Here's how the part is built. I have some questions about the finished solid (model axes, mm). Give positions to 0.01 mm unless a question says otherwise; leave off trailing zeros. Loops run counter-clockwise (first coordinate to the right, second up) from the corner with the lowest first, then second, coordinate; pieces in that order, holes last.
Q1. If we section it at A-A (z = -1.7): Please give me the cut outline in (x, y) (1 decimal), plus the area to 3 significant figures.
Q2. I need wall thicknesses on line 1 (Y direction, x = 10, z = -2.2); line 2 (X direction, y = 135.25, z = -1.4); line 3 (Y direction, x = 31.5, z = -3). Which ranges of each line are inside material? Lowest first, please.
Q3. If we section it at C-C (x = 140.5): Please give me the cut outline in (y, z) (3 decimals).
Q4. If we section it at B-B (x = 26.5): Please give me the cut outline in (y, z) (3 decimals).
from build123d import *

# Parameters (mm, degrees)
SKETCH1_R           = 0.635
BOSS_EXTRUDE1_DEPTH = 3.175


with BuildPart() as part:
    # Sketch1 → Boss-Extrude1 (new body)
    with BuildSketch(Plane.XY):
        Polygon((1.5875, 128.192969627), (1.5875, 141.955116052), (169.8625, 140.597136541), (169.8625, 127.291804233), align=None)
        with Locations((10.495441348, 135.01829257)):
            Circle(SKETCH1_R, mode=Mode.SUBTRACT)
    extrude(amount=-BOSS_EXTRUDE1_DEPTH)


solid = part.part
Check sheet entries:
1. outline: (1.6, 128.2) - (169.9, 127.3) - (169.9, 140.6) - (1.6, 142) - close; hole circle Ø1.3 at (10.5, 135)
1. area: 2,280 mm2
2. line 1: y = 128.15 to 134.62, 135.42 to 141.89
2. line 2: x = 1.59 to 9.9, 11.09 to 169.86
2. line 3: y = 128.03 to 141.71
3. outline: (127.449, -3.175) - (140.834, -3.175) - (140.834, 0) - (127.449, 0) - close
4. outline: (128.06, -3.175) - (141.754, -3.175) - (141.754, 0) - (128.06, 0) - close
